from build123d import *

# Parameters (mm, degrees)
EXTRUDE_1_DEPTH     = 20
SKETCH_2_R          = 2.5
CUT_EXTRUDE_1_DEPTH = 20
FILLET_1_R          = 10
CHAMFER_1_SIZE      = 4
CHAMFER_2_SIZE      = 2
FILLET_2_R          = 3
CHAMFER_3_SIZE      = 0.4


with BuildPart() as part:
    # 草图1 → 凸台-拉伸1 (new body)
    with BuildSketch(Plane(origin=(0, 0, 0), x_dir=(1, 0, 0), z_dir=(0, 1, 0))):
        Polygon((0, 0), (4, 0), (4, 21), (34, 21), (34, 25), (4, 25), (0, 25), align=None)
    extrude(amount=EXTRUDE_1_DEPTH)

    # 草图2 → 切除-拉伸1 (cut)
    with BuildSketch(Plane(origin=(4, 0, 0), x_dir=(0, 0, -1), z_dir=(1, 0, 0))):
        with Locations((10.5, 10)):
            Circle(SKETCH_2_R)
    extrude(amount=-CUT_EXTRUDE_1_DEPTH, mode=Mode.SUBTRACT)

    # 圆角1
    fillet_1_edges = [part.edges().sort_by_distance(p)[0] for p in [
        (2, 0, 0),
        (2, 20, 0),
    ]]
    fillet(fillet_1_edges, radius=FILLET_1_R - 0.0001)  # a hair under: the kernel refuses the full size

    # 倒角1
    chamfer_1_edges = [part.edges().sort_by_distance(p)[0] for p in [
        (4, 10, -21),
    ]]
    chamfer(chamfer_1_edges, length=CHAMFER_1_SIZE)

    # 倒角2
    chamfer_2_edges = [part.edges().sort_by_distance(p)[0] for p in [
        (0, 10, -25),
    ]]
    chamfer(chamfer_2_edges, length=CHAMFER_2_SIZE)

    # 圆角2
    fillet_2_edges = [part.edges().sort_by_distance(p)[0] for p in [
        (34, 20, -23),
        (34, 0, -23),
    ]]
    fillet(fillet_2_edges, radius=FILLET_2_R)

    # 倒角3
    chamfer_3_edges = [part.edges().sort_by_distance(p)[0] for p in [
        (4, 0, -13.49995),
        (4, 20, -13.49995),
        (4, 17.071097101, -2.928902899),
        (4, 2.928902899, -2.928902899),
        (0, 17.071097101, -2.928902899),
        (0, 2.928902899, -2.928902899),
        (19.5, 0, -21),
        (19.5, 20, -21),
        (6, 0, -19),
        (6, 20, -19),
        (0, 0, -16.49995),
        (0, 20, -16.49995),
        (1, 0, -24),
        (1, 20, -24),
        (34, 10, -25),
        (34, 10, -21),
        (16.5, 0, -25),
        (16.5, 20, -25),
        (33.121320344, 19.121320344, -25),
        (33.121320344, 0.878679656, -25),
        (33.121320344, 19.121320344, -21),
        (33.121320344, 0.878679656, -21),
    ]]
    chamfer(chamfer_3_edges, length=CHAMFER_3_SIZE)


solid = part.part
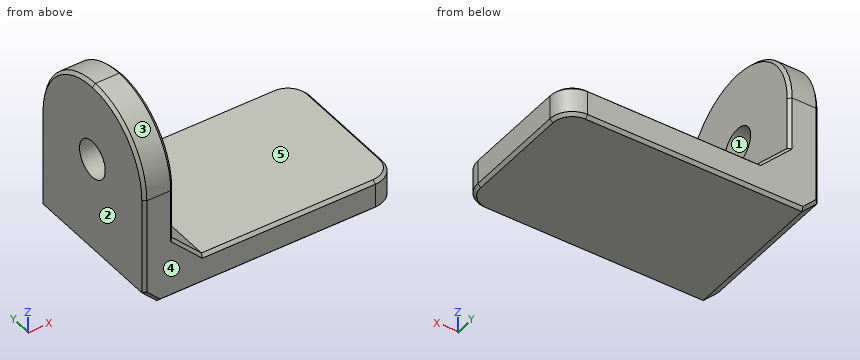
Here's how the part is built. I have some questions about the finished solid (model axes, mm). Face numbers are marked on the shaded views. A direction names the side the tool comes from. Coordinates: 2 decimals unless noted, no trailing zeros. Write each loop counter-clockwise with the first axis right and the second up, starting at its lowest first coordinate (ties: lowest second). Pieces come first, ordered by that corner, then holes.
Item 1: If I drill on line 1 (Y direction, x = 1.15, z = -10.5); line 2 (X direction, y = 1.5, z = -12.25); line 3 (Z direction, x = 10, y = 2.25), over which ranges is the centre line in solid material (lowest first)?
Item 2: I want a section at C-C on z = -14. Write out the boundary of the cut face in (x, y), and give its area (3 significant figures).
Item 3: If we mould it in two halves opening along Z, with no side actions, what happens to the marked faces 1, 2 and 3? For each: +Z half, -Z half, draft (parallel to the pull), parting line (faces both ways), or undercut.
Item 4: I want a section at B-B on x = 28. Write out the boundary of the cut face in (y, z), and give its area (3 significant figures).
Item 5: I want a section at A-A on z = -10.5. Write out the boundary of the cut face in (x, y), and give its area (3 significant figures).
Item 6: On a 3-axis mill with a long thin cutter (end or side, diameter ignored), from which of +Z, -Z, +X, -X, +Y, -Y can I reach the whole of each face in a straight line? I mean the marked faces 4 and 5. Say none if no direction works.
Item 7: Will these pins go through, and if not, where does the flat tip stop? pin 1 (10 mm diameter, centred on x = 10.5, y = 11, fed in from +Z); pin 2 (12 mm diameter, centred on y = 5.5, z = -7.5, fed in from +X); pin 3 (8 mm diameter, centred on x = 28.5, y = 12.5, fed in from +Z).
Findings below:
1. line 1: y = 0 to 7.5, 12.5 to 20
1. line 2: x = 0 to 4
1. line 3: z = -25 to -21
2. outline: (0, 0.4) - (0.4, 0) - (3.6, 0) - (4, 0.4) - (4, 19.6) - (3.6, 20) - (0.4, 20) - (0, 19.6) - close
2. area: 79.7 mm2
3. face 1: undercut
3. face 2: draft
3. face 3: +Z half
4. outline: (0, -24.6) - (0.4, -25) - (19.6, -25) - (20, -24.6) - (20, -21.4) - (19.6, -21) - (0.4, -21) - (0, -21.4) - close
4. area: 79.7 mm2
5. outline: (0, 0.4) - (0.4, 0) - (3.6, 0) - (4, 0.4) - (4, 7.5) - (0, 7.5) - close; (0, 12.5) - (4, 12.5) - (4, 19.6) - (3.6, 20) - (0.4, 20) - (0, 19.6) - close
5. area: 59.7 mm2
6. face 4: +Z, -Z, +X, -X, -Y
6. face 5: +Z, +X, +Y, -Y
7. pin 1: stops at z = -18.5
7. pin 2: stops at x = 4
7. pin 3: stops at z = -21
